```python
from build123d import *

# Parameters (mm, degrees)
SKETCH1_R                                      = 26.8
BOSS_EXTRUDE1_DEPTH                            = 6
CBORE_FOR_8_SOCKET_HEAD_CAP_SCREW1_D           = 4.4958
CBORE_FOR_8_SOCKET_HEAD_CAP_SCREW1_DEPTH       = 11.043366656
CBORE_FOR_8_SOCKET_HEAD_CAP_SCREW1_CBORE_D     = 7.9375
CBORE_FOR_8_SOCKET_HEAD_CAP_SCREW1_CBORE_DEPTH = 4.1656
SKETCH3_W                                      = 37.2978219
SKETCH3_H                                      = 2
CUT_EXTRUDE1_DEPTH                             = 12
BOSS_EXTRUDE2_DEPTH                            = 12
F_8_32_TAPPED_HOLE1_D                          = 3.4544
F_8_CLEARANCE_HOLE1_D                          = 4.9149
F_8_CLEARANCE_HOLE1_DEPTH                      = 4
F_8_CLEARANCE_HOLE1_TIP                        = 1.476584928


with BuildPart() as part:
    # Sketch1 → Boss-Extrude1 (new, symmetric)
    with BuildSketch(Plane(origin=(0, 0, 0), x_dir=(1, 0, 0), z_dir=(0, 1, 0))):
        with BuildLine():
            Line((6.5, -31.843366656), (6.5, -37.843366656))
            Line((6.5, -37.843366656), (-6.5, -37.843366656))
            Line((-6.5, -37.843366656), (-6.5, -31.843366656))
            ThreePointArc((-6.5, -31.843366656), (0, 32.5), (6.5, -31.843366656))
        make_face()
        with Locations(Location((0, 0, 0), (0, 0, 270))):
            Circle(SKETCH1_R, mode=Mode.SUBTRACT)
    extrude(amount=BOSS_EXTRUDE1_DEPTH, both=True)

    # CBORE for #8 Socket Head Cap Screw1
    with Locations(Plane(origin=(0, 0, 26.8), x_dir=(-1, 0, 0), z_dir=(0, 0, -1))):
        with Locations((0, 0)):
            CounterBoreHole(CBORE_FOR_8_SOCKET_HEAD_CAP_SCREW1_D / 2, CBORE_FOR_8_SOCKET_HEAD_CAP_SCREW1_CBORE_D / 2, CBORE_FOR_8_SOCKET_HEAD_CAP_SCREW1_CBORE_DEPTH, depth=CBORE_FOR_8_SOCKET_HEAD_CAP_SCREW1_DEPTH)

    # Sketch3 → Cut-Extrude1 (cut)
    with BuildSketch(Plane(origin=(0, 6, 0), x_dir=(1, 0, 0), z_dir=(0, 1, 0))):
        with Locations((-18.64891095, 0)):
            Rectangle(SKETCH3_W, SKETCH3_H)
    extrude(amount=-CUT_EXTRUDE1_DEPTH, mode=Mode.SUBTRACT)

    # Sketch4 → Boss-Extrude2 (add)
    with BuildSketch(Plane(origin=(0, 6, 0), x_dir=(1, 0, 0), z_dir=(0, 1, 0))):
        with BuildLine():
            Line((-32.484611742, -1), (-42.113081447, -1))
            Line((-42.113081447, -1), (-42.113081447, -5))
            Line((-42.113081447, -5), (-32.113081447, -5))
            ThreePointArc((-32.113081447, -5), (-32.360709067, -3.005745946), (-32.484611742, -1))
        make_face()
        with BuildLine():
            Line((-32.484611742, 1), (-42.113081447, 1))
            Line((-42.113081447, 1), (-42.113081447, 5))
            Line((-42.113081447, 5), (-32.113081447, 5))
            ThreePointArc((-32.113081447, 5), (-32.360709067, 3.005745946), (-32.484611742, 1))
        make_face()
    extrude(amount=-BOSS_EXTRUDE2_DEPTH)

    # #8-32 Tapped Hole1 (through all)
    with Locations(Plane(origin=(0, 0, -5), x_dir=(-1, 0, 0), z_dir=(0, 0, -1))):
        with Locations((36.885640573, 0)):
            Hole(F_8_32_TAPPED_HOLE1_D / 2)

    # #8 Clearance Hole1
    with Locations(Plane(origin=(0, 0, -5), x_dir=(-1, 0, 0), z_dir=(0, 0, -1))):
        with Locations((36.885640573, 0)):
            Hole(F_8_CLEARANCE_HOLE1_D / 2, depth=F_8_CLEARANCE_HOLE1_DEPTH)
            with Locations((0, 0, -(F_8_CLEARANCE_HOLE1_DEPTH + F_8_CLEARANCE_HOLE1_TIP / 2))):  # 118° drill point
                Cone(0, F_8_CLEARANCE_HOLE1_D / 2, F_8_CLEARANCE_HOLE1_TIP, mode=Mode.SUBTRACT)


solid = part.part
```
For this review, take the finished solid that the model builds, in its own axes (mm). A direction names the side the tool comes from. Round coordinates to 2 decimals unless told otherwise and drop trailing zeros. Write each loop counter-clockwise with the first axis right and the second up, starting at its lowest first coordinate (ties: lowest second). Pieces come first, ordered by that corner, then holes. Notation, with made-up numbers: (-32.75, 22.25) -> (7.25, 22.25) arc R25 ccw to (7.25, 45.25) -> close; hole circle Ø11 at (37.25, 72). An arc over 180 degrees is marked (long way). Use one line per item in the form item = value.
1) Mouldability with a two-part tool opening along Y and no side actions: class faces 1 (the flat face through (-8, 6, 26)), 2 (the cylindrical face through (-34.542, 0.738, -2.972)), 3 (the flat face through (-34.6, 1.4, -1)) as +Y half, -Y half, draft (parallel to the pull), parting line (faces both ways), or undercut.
Found:
face_1 = +Y half
face_2 = undercut
face_3 = draft
2) Take a section at A-A, the plane z = 13. Write out the cut boundary in (x, y).
Found:
outline = (-29.79, -6) -> (-23.44, -6) -> (-23.44, 6) -> (-29.79, 6) -> close; (23.44, -6) -> (29.79, -6) -> (29.79, 6) -> (23.44, 6) -> close
3) Tool access review of faces 4 (the flat face through (-34, 0, 1)), 5 (the cylindrical face through (2.076, -0.861, 34.453)), 6 (the flat face through (-2, -2, 30.966)): name each direction out of +Z, -Z, +X, -X, +Y, -Y from which nothing blocks a thin tool from reaching the whole face with its end or side.
Found:
face_4 = -X, +Y, -Y
face_5 = +Z
face_6 = none
4) Take a section at B-B, the plane x = -15. Write out the cut boundary in (y, z), and give its area (3 significant figures).
Found:
outline = (-6, -28.83) -> (6, -28.83) -> (6, -22.21) -> (-6, -22.21) -> close; (-6, 22.21) -> (6, 22.21) -> (6, 28.83) -> (-6, 28.83) -> close
area = 159 mm2
5) Take a section at D-D, the plane z = 0. Write out the cut boundary in (x, y), and give its area (3 significant figures).
Found:
outline = (26.8, -6) -> (32.5, -6) -> (32.5, 6) -> (26.8, 6) -> close
area = 68.4 mm2
6) Clearance check with flat-ended pins moving along their axes: pin 1 (4 mm diameter, centred on x = 17.5, y = 1, fed in from +Z); pin 2 (2 mm diameter, centred on x = 4, y = -3.5, fed in from -Z); pin 3 (3 mm diameter, centred on y = 2, z = 36.5, fed in from +X). State where each tip first meets the part, or that it passes through.
Found:
pin_1 = 28.57
pin_2 = -32.36
pin_3 = 6.5
7) Take a section at C-C, the plane x = -37. Write out the cut boundary in (y, z).
Found:
outline = (-6, -5) -> (-2.45, -5) -> (-2.45, -1) -> (-6, -1) -> close; (-6, 1) -> (-1.72, 1) -> (-1.72, 5) -> (-6, 5) -> close; (1.72, 1) -> (6, 1) -> (6, 5) -> (1.72, 5) -> close; (2.45, -5) -> (6, -5) -> (6, -1) -> (2.45, -1) -> close
8) To check wall thickness, follow L1, parallel to Z at x = -1, y = -2.75; L2, parallel to X at y = 0, z = -3; L3, parallel to X at y = -1.5, z = 19.5. State the ranges of each line that lie inside material, in increasing order. Write a range as from..to.
Found:
L1 = -32.48..-26.78, 30.97..37.84
L2 = -42.11..-39.34, -34.43..-26.63, 26.63..32.36
L3 = -26..-18.38, 18.38..26
